Could you check a few things on this model? Use its own coordinates, in mm. Round coordinates to 2 decimals unless told otherwise and drop trailing zeros. Order: outer loops, then holes, each group sorted by start corner. A loop starts at its lowest first (then second) coordinate and runs counter-clockwise, first axis right, second up. Notation, with made-up numbers: M -9.75,-20.5 L 28.25,-20.5 A35 cw 28.25,16.5 Z; hole C 76.25,43.5 d5. An arc over 180 degrees is marked long. Write each question's results on one line, items separated by ' | '. Start each with the question number.
1. I'm going to push flat-ended pins straight in: pin 1 (4.5 mm diameter, centred on x = 232.41, z = -9.525, fed in from +Y); pin 2 (9 mm diameter, centred on x = 73.406, z = -9.525, fed in from -Y). Where does each tip first touch, or does it pass through?
2. Suppose I cut it at B-B on z = -10. Give the number of separate pieces and of enclosed holes in the cut face, and give its area (3 significant figures).
3. Please list where these lines run through material, in increasing order: L1, parallel to Z at x = 232.41, y = 1.85; L2, parallel to Z at x = 201, y = 1.7; L3, parallel to Y at x = 103, z = -12.
4. Suppose I cut it at A-A on x = 232.41. Write out the boundary of the cut face in (y, z).
5. We'd pull the mould along Z, two halves only. Please class faces 1 (the flat face through (120, 0, -10)), 2 (the conical face through (136.534, 1.638, -9.143)): released by +Z, released by -Z, zero draft, split by the parting line, or undercut.
from build123d import *

# Parameters (mm, degrees)
SKETCH1_W                                  = 243.84
SKETCH1_H                                  = 19.05
BOSS_EXTRUDE1_DEPTH                        = 2.032
CSK_FOR_10_FLAT_HEAD_MACHINE_SCREW_2_COUNT = 2
CSK_FOR_10_FLAT_HEAD_MACHINE_SCREW_2_PITCH = 30.988
CSK_FOR_10_FLAT_HEAD_MACHINE_SCREW_3_COUNT = 2
CSK_FOR_10_FLAT_HEAD_MACHINE_SCREW_3_PITCH = 61.976
CSK_FOR_10_FLAT_HEAD_MACHINE_SCREW_4_COUNT = 2
CSK_FOR_10_FLAT_HEAD_MACHINE_SCREW_4_PITCH = 92.964
CSK_FOR_10_FLAT_HEAD_MACHINE_SCREW_5_COUNT = 2
CSK_FOR_10_FLAT_HEAD_MACHINE_SCREW_5_PITCH = 128.016
CSK_FOR_10_FLAT_HEAD_MACHINE_SCREW_6_COUNT = 2
CSK_FOR_10_FLAT_HEAD_MACHINE_SCREW_6_PITCH = 159.004
CSK_FOR_10_FLAT_HEAD_MACHINE_SCREW_7_COUNT = 2
CSK_FOR_10_FLAT_HEAD_MACHINE_SCREW_7_PITCH = 189.992
CSK_FOR_10_FLAT_HEAD_MACHINE_SCREW_8_COUNT = 2
CSK_FOR_10_FLAT_HEAD_MACHINE_SCREW_8_PITCH = 220.98


with BuildPart() as part:
    # Sketch1 → Boss-Extrude1 (new body)
    with BuildSketch(Plane(origin=(0, 0, 0), x_dir=(1, 0, 0), z_dir=(0, 1, 0))):
        with Locations((121.92, 9.525)):
            Rectangle(SKETCH1_W, SKETCH1_H)
    extrude(amount=BOSS_EXTRUDE1_DEPTH)

    # Sketch3 → CSK for #10 Flat Head Machine Screw (100)1 (revolve, cut)
    with BuildSketch(Plane(origin=(11.43, 0, -9.525), x_dir=(0, 0, -1), z_dir=(1, 0, 0))):
        Polygon((0, 0), (0, 2.032), (2.8067, 2.032), (2.8067, 1.747676712), (4.8895, 0), align=None)
    csk_for_10_flat_head_machine_screw_100 = revolve(axis=Axis((11.43, -6.35, -9.525), (0, 1, 0)), mode=Mode.SUBTRACT)

    # CSK for _10 Flat Head Machine Screw  2: CSK for #10 Flat Head Machine Screw (100)1 ×2
    with Locations(*[(i * CSK_FOR_10_FLAT_HEAD_MACHINE_SCREW_2_PITCH, 0, 0) for i in range(1, CSK_FOR_10_FLAT_HEAD_MACHINE_SCREW_2_COUNT)]):
        add(csk_for_10_flat_head_machine_screw_100, mode=Mode.SUBTRACT)

    # CSK for _10 Flat Head Machine Screw  3: CSK for #10 Flat Head Machine Screw (100)1 ×2
    with Locations(*[(i * CSK_FOR_10_FLAT_HEAD_MACHINE_SCREW_3_PITCH, 0, 0) for i in range(1, CSK_FOR_10_FLAT_HEAD_MACHINE_SCREW_3_COUNT)]):
        add(csk_for_10_flat_head_machine_screw_100, mode=Mode.SUBTRACT)

    # CSK for _10 Flat Head Machine Screw  4: CSK for #10 Flat Head Machine Screw (100)1 ×2
    with Locations(*[(i * CSK_FOR_10_FLAT_HEAD_MACHINE_SCREW_4_PITCH, 0, 0) for i in range(1, CSK_FOR_10_FLAT_HEAD_MACHINE_SCREW_4_COUNT)]):
        add(csk_for_10_flat_head_machine_screw_100, mode=Mode.SUBTRACT)

    # CSK for _10 Flat Head Machine Screw  5: CSK for #10 Flat Head Machine Screw (100)1 ×2
    with Locations(*[(i * CSK_FOR_10_FLAT_HEAD_MACHINE_SCREW_5_PITCH, 0, 0) for i in range(1, CSK_FOR_10_FLAT_HEAD_MACHINE_SCREW_5_COUNT)]):
        add(csk_for_10_flat_head_machine_screw_100, mode=Mode.SUBTRACT)

    # CSK for _10 Flat Head Machine Screw  6: CSK for #10 Flat Head Machine Screw (100)1 ×2
    with Locations(*[(i * CSK_FOR_10_FLAT_HEAD_MACHINE_SCREW_6_PITCH, 0, 0) for i in range(1, CSK_FOR_10_FLAT_HEAD_MACHINE_SCREW_6_COUNT)]):
        add(csk_for_10_flat_head_machine_screw_100, mode=Mode.SUBTRACT)

    # CSK for _10 Flat Head Machine Screw  7: CSK for #10 Flat Head Machine Screw (100)1 ×2
    with Locations(*[(i * CSK_FOR_10_FLAT_HEAD_MACHINE_SCREW_7_PITCH, 0, 0) for i in range(1, CSK_FOR_10_FLAT_HEAD_MACHINE_SCREW_7_COUNT)]):
        add(csk_for_10_flat_head_machine_screw_100, mode=Mode.SUBTRACT)

    # CSK for _10 Flat Head Machine Screw  8: CSK for #10 Flat Head Machine Screw (100)1 ×2
    with Locations(*[(i * CSK_FOR_10_FLAT_HEAD_MACHINE_SCREW_8_PITCH, 0, 0) for i in range(1, CSK_FOR_10_FLAT_HEAD_MACHINE_SCREW_8_COUNT)]):
        add(csk_for_10_flat_head_machine_screw_100, mode=Mode.SUBTRACT)


solid = part.part
Filled sheet:
1) pin 1: passes through | pin 2: stops at y = 0.33
2) separate pieces: 9 | enclosed holes: 0 | area: 376 mm^2
3) L1: z = -19.05 to -12.33, -6.72 to 0 | L2: z = -19.05 to -12.36, -6.69 to 0 | L3: y = 1.72 to 2.03
4) outline: M 0,-19.05 L 2.03,-19.05 L 2.03,-12.33 L 1.75,-12.33 L 0,-14.41 Z; M 0,-4.64 L 1.75,-6.72 L 2.03,-6.72 L 2.03,0 L 0,0 Z
5) face 1: zero draft | face 2: undercut
